from build123d import *

# Parameters (mm, degrees)
SKETCH_1_W          = 180
SKETCH_1_H          = 94
EXTRUDE_1_DEPTH     = 3
SKETCH_2_W          = 6
SKETCH_2_H          = 10
SKETCH_2_H_2        = 33.9
SKETCH_2_H_3        = 32.9
SKETCH_2_W_2        = 10
SKETCH_2_H_4        = 8
EXTRUDE_2_DEPTH     = 9
CHAMFER_2_SIZE      = 6
CHAMFER_1_SIZE      = 6
CUT_EXTRUDE_1_REACH = 205.421
SKETCH_3_R          = 1.5
SKETCH_3_R_2        = 1.75
SKETCH_4_R          = 1.5
CUT_EXTRUDE_2_DEPTH = 204.265835791
SKETCH_5_W          = 4
SKETCH_5_H          = 46
EXTRUDE_3_DEPTH     = 4
CHAMFER_3_SIZE      = 2
SKETCH_6_W          = 12
SKETCH_6_H          = 19.9
EXTRUDE_4_DEPTH     = 4
FILLET_1_R          = 4
SKETCH_7_W          = 12
SKETCH_7_H          = 19.9
EXTRUDE_5_DEPTH     = 4
FILLET_2_R          = 4
FILLET_3_R          = 2
SKETCH_8_R          = 1.5
CUT_EXTRUDE_3_DEPTH = 10
CUT_EXTRUDE_4_REACH = 208.969
SKETCH_9_R          = 1.5
CHAMFER_4_SIZE      = 6
FILLET_4_R          = 2


with BuildPart() as part:
    # Эскиз1 → Бобышка-Вытянуть1 (new body)
    with BuildSketch(Plane.XY):
        with Locations((90, -47)):
            Rectangle(SKETCH_1_W, SKETCH_1_H)
    extrude(amount=EXTRUDE_1_DEPTH)

    # Эскиз2 → Бобышка-Вытянуть2 (add)
    with BuildSketch(Plane.XY.offset(3)):
        with Locations((3, -89)):
            Rectangle(SKETCH_2_W, SKETCH_2_H)
        with Locations((177, -89)):
            Rectangle(SKETCH_2_W, SKETCH_2_H)
        with Locations((3, -52)):
            Rectangle(SKETCH_2_W, SKETCH_2_H)
        with Locations((177, -53)):
            Rectangle(SKETCH_2_W, SKETCH_2_H)
        with Locations((177, -25.05)):
            Rectangle(SKETCH_2_W, SKETCH_2_H_2)
        with Locations((3, -24.55)):
            Rectangle(SKETCH_2_W, SKETCH_2_H_3)
        with Locations((90.875995779, -90)):
            Rectangle(SKETCH_2_W_2, SKETCH_2_H_4)
    extrude(amount=EXTRUDE_2_DEPTH)

    # Фаска2
    chamfer_2_edges = [part.edges().sort_by_distance(p)[0] for p in [
        (3, -57, 3),
        (177, -58, 3),
    ]]
    chamfer(chamfer_2_edges, length=CHAMFER_2_SIZE)

    # Фаска1
    chamfer_1_edges = [part.edges().sort_by_distance(p)[0] for p in [
        (3, -84, 3),
        (177, -84, 3),
    ]]
    chamfer(chamfer_1_edges, length=CHAMFER_1_SIZE)

    # Эскиз3 → Вырез-Вытянуть1 (cut, up to next)
    with BuildSketch(Plane(origin=(180, 0, 0), x_dir=(0, 0, -1), z_dir=(1, 0, 0)), mode=Mode.PRIVATE) as cut_extrude_1_sk1:
        with Locations((-6, -89)):
            Circle(SKETCH_3_R)
    cut_extrude_1_tool1 = extrude(cut_extrude_1_sk1.sketch, amount=-CUT_EXTRUDE_1_REACH, mode=Mode.PRIVATE) & part.part
    # Эскиз3 → Вырез-Вытянуть1 (cut, up to next)
    with BuildSketch(Plane(origin=(180, 0, 0), x_dir=(0, 0, -1), z_dir=(1, 0, 0)), mode=Mode.PRIVATE) as cut_extrude_1_sk2:
        with Locations((-6, -53)):
            Circle(SKETCH_3_R)
    cut_extrude_1_tool2 = extrude(cut_extrude_1_sk2.sketch, amount=-CUT_EXTRUDE_1_REACH, mode=Mode.PRIVATE) & part.part
    # Эскиз3 → Вырез-Вытянуть1 (cut, up to next)
    with BuildSketch(Plane(origin=(180, 0, 0), x_dir=(0, 0, -1), z_dir=(1, 0, 0)), mode=Mode.PRIVATE) as cut_extrude_1_sk3:
        with Locations((-6, -34)):
            Circle(SKETCH_3_R_2)
    cut_extrude_1_tool3 = extrude(cut_extrude_1_sk3.sketch, amount=-CUT_EXTRUDE_1_REACH, mode=Mode.PRIVATE) & part.part
    add(cut_extrude_1_tool1.solids().sort_by_distance((180, -89, 6))[0], mode=Mode.SUBTRACT)
    add(cut_extrude_1_tool2.solids().sort_by_distance((180, -53, 6))[0], mode=Mode.SUBTRACT)
    add(cut_extrude_1_tool3.solids().sort_by_distance((180, -34, 6))[0], mode=Mode.SUBTRACT)

    # Эскиз4 → Вырез-Вытянуть2 (cut, through all)
    with BuildSketch(Plane.XY.offset(3)):
        with Locations((4, -4)):
            Circle(SKETCH_4_R)
        with Locations((176, -4)):
            Circle(SKETCH_4_R)
        with Locations((58, -4)):
            Circle(SKETCH_4_R)
        with Locations((122, -4)):
            Circle(SKETCH_4_R)
    extrude(amount=-CUT_EXTRUDE_2_DEPTH, mode=Mode.SUBTRACT)

    # Эскиз5 → Бобышка-Вытянуть3 (add)
    with BuildSketch(Plane.XY.offset(3)):
        with Locations((42, -71)):
            Rectangle(SKETCH_5_W, SKETCH_5_H)
        with Locations((138, -71)):
            Rectangle(SKETCH_5_W, SKETCH_5_H)
        Polygon((27, -4.5), (27, -37), (6, -37), (6, -41), (174, -41), (174, -37), (153, -37), (153, -4.5), (149, -4.5), (149, -37), (94, -37), (94, -4.5), (86, -4.5), (86, -37), (31, -37), (31, -4.5), align=None)
    extrude(amount=EXTRUDE_3_DEPTH)

    # Фаска3
    # the kernel refuses this chamfer: 2 mm, written as the material it adds along each edge
    with BuildSketch(Plane(origin=(6, -72.856634024, 3), x_dir=(0.9996219169112968, 0, -0.02749587661058627), z_dir=(0, -1, 0))) as chamfer_3_piece_1_section:
        Polygon((CHAMFER_3_SIZE * 0.999621916911, CHAMFER_3_SIZE * 0.0274958766106), (-CHAMFER_3_SIZE * 0.0274958766106, CHAMFER_3_SIZE * 0.999621916911), (0, 0), align=None)
    chamfer_3_piece_1 = extrude(amount=21.143365976, mode=Mode.PRIVATE)
    chamfer_3_piece_1 = split(chamfer_3_piece_1, bisect_by=Plane(origin=(6.668439358, -82.482271763, 7.482271763), z_dir=(0, -0.7071067811865476, -0.7071067811865476)), keep=Keep.TOP, mode=Mode.PRIVATE)
    add(chamfer_3_piece_1)
    with BuildSketch(Plane(origin=(174, -94, 3), x_dir=(-0.9996219169112968, 0, -0.02749587661058639), z_dir=(0, 1, 0))) as chamfer_3_piece_2_section:
        Polygon((CHAMFER_3_SIZE * 0.999621916911, CHAMFER_3_SIZE * 0.0274958766106), (-CHAMFER_3_SIZE * 0.0274958766106, CHAMFER_3_SIZE * 0.999621916911), (0, 0), align=None)
    chamfer_3_piece_2 = extrude(amount=21.143365976, mode=Mode.PRIVATE)
    chamfer_3_piece_2 = split(chamfer_3_piece_2, bisect_by=Plane(origin=(173.327651835, -82.469530213, 7.469530213), z_dir=(2.038461385028344e-15, -0.7071067811865476, -0.7071067811865476)), keep=Keep.TOP, mode=Mode.PRIVATE)
    chamfer_3_piece_2 = chamfer_3_piece_2 - Plane(origin=(173.327651835, -89, 6), x_dir=(0, 0, -1), z_dir=(1, 0, 0)) * Cylinder(1.5, 51, mode=Mode.PRIVATE)
    add(chamfer_3_piece_2)
    with BuildSketch(Plane(origin=(6, -47, 3), x_dir=(0.9996219169112968, 0, -0.02749587661058627), z_dir=(0, -1, 0))) as chamfer_3_piece_3_section:
        Polygon((CHAMFER_3_SIZE * 0.999621916911, CHAMFER_3_SIZE * 0.0274958766106), (-CHAMFER_3_SIZE * 0.0274958766106, CHAMFER_3_SIZE * 0.999621916911), (0, 0), align=None)
    chamfer_3_piece_3 = extrude(amount=21.143365976, mode=Mode.PRIVATE)
    chamfer_3_piece_3 = split(chamfer_3_piece_3, bisect_by=Plane(origin=(6.668439358, -58.517728237, 7.482271763), z_dir=(0, 0.7071067811865476, -0.7071067811865476)), keep=Keep.TOP, mode=Mode.PRIVATE)
    add(chamfer_3_piece_3)
    with BuildSketch(Plane(origin=(174, -69.143365976, 3), x_dir=(-0.9996219169112968, 0, -0.02749587661058639), z_dir=(0, 1, 0))) as chamfer_3_piece_4_section:
        Polygon((CHAMFER_3_SIZE * 0.999621916911, CHAMFER_3_SIZE * 0.0274958766106), (-CHAMFER_3_SIZE * 0.0274958766106, CHAMFER_3_SIZE * 0.999621916911), (0, 0), align=None)
    chamfer_3_piece_4 = extrude(amount=21.143365976, mode=Mode.PRIVATE)
    chamfer_3_piece_4 = split(chamfer_3_piece_4, bisect_by=Plane(origin=(173.327651834, -59.530469789, 7.469530211), z_dir=(0, 0.7071067811865476, -0.7071067811865476)), keep=Keep.TOP, mode=Mode.PRIVATE)
    chamfer_3_piece_4 = chamfer_3_piece_4 - Plane(origin=(173.327651834, -53, 6), x_dir=(0, 0, -1), z_dir=(1, 0, 0)) * Cylinder(1.5, 51, mode=Mode.PRIVATE)
    add(chamfer_3_piece_4)

    # Эскиз6 → Бобышка-Вытянуть4 (add)
    with BuildSketch(Plane(origin=(180, 0, 0), x_dir=(0, 0, -1), z_dir=(1, 0, 0))):
        with Locations((-6, -18.05)):
            Rectangle(SKETCH_6_W, SKETCH_6_H)
    extrude(amount=EXTRUDE_4_DEPTH)

    # Скругление1
    fillet_1_edges = [part.edges().sort_by_distance(p)[0] for p in [
        (184, -18.05, 12),
    ]]
    fillet(fillet_1_edges, radius=FILLET_1_R)

    # Эскиз7 → Бобышка-Вытянуть5 (add)
    with BuildSketch(Plane.ZY):
        with Locations((6, -18.05)):
            Rectangle(SKETCH_7_W, SKETCH_7_H)
    extrude(amount=EXTRUDE_5_DEPTH)

    # Скругление2
    fillet_2_edges = [part.edges().sort_by_distance(p)[0] for p in [
        (-4, -18.05, 12),
    ]]
    fillet(fillet_2_edges, radius=FILLET_2_R)

    # Скругление3
    fillet_3_edges = [part.edges().sort_by_distance(p)[0] for p in [
        (184, -18.05, 0),
        (-4, -18.05, 0),
    ]]
    fillet(fillet_3_edges, radius=FILLET_3_R)

    # Эскиз8 → Вырез-Вытянуть3 (cut)
    with BuildSketch(Plane.XZ.offset(94)):
        with Locations(Location((90.875995779, 8, 0), (0, 0, 270))):
            Circle(SKETCH_8_R)
    extrude(amount=-CUT_EXTRUDE_3_DEPTH, mode=Mode.SUBTRACT)

    # Эскиз9 → Вырез-Вытянуть4 (cut, up to next)
    with BuildSketch(Plane.ZY, mode=Mode.PRIVATE) as cut_extrude_4_sk1:
        with Locations(Location((6, -89, 0), (0, 0, 180))):
            Circle(SKETCH_9_R)
    cut_extrude_4_tool1 = extrude(cut_extrude_4_sk1.sketch, amount=-CUT_EXTRUDE_4_REACH, mode=Mode.PRIVATE) & part.part
    # Эскиз9 → Вырез-Вытянуть4 (cut, up to next)
    with BuildSketch(Plane.ZY, mode=Mode.PRIVATE) as cut_extrude_4_sk2:
        with Locations(Location((6, -53, 0), (0, 0, 180))):
            Circle(SKETCH_9_R)
    cut_extrude_4_tool2 = extrude(cut_extrude_4_sk2.sketch, amount=-CUT_EXTRUDE_4_REACH, mode=Mode.PRIVATE) & part.part
    add(cut_extrude_4_tool1.solids().sort_by_distance((0, -89, 6))[0], mode=Mode.SUBTRACT)
    add(cut_extrude_4_tool2.solids().sort_by_distance((0, -53, 6))[0], mode=Mode.SUBTRACT)

    # Фаска4
    chamfer_4_edges = [part.edges().sort_by_distance(p)[0] for p in [
        (85.875995779, -90, 3),
        (95.875995779, -90, 3),
    ]]
    chamfer(chamfer_4_edges, length=CHAMFER_4_SIZE)

    # Скругление4
    fillet_4_edges = [part.edges().sort_by_distance(p)[0] for p in [
        (177, -84, 12),
        (3, -84, 12),
        (3, -41, 12),
        (3, -47, 12),
        (3, -57, 12),
        (3, -94, 12),
        (177, -42, 12),
        (177, -48, 12),
        (177, -58, 12),
        (85.875995779, -90, 12),
        (95.875995779, -90, 12),
        (177, -94, 12),
    ]]
    fillet(fillet_4_edges, radius=FILLET_4_R)


solid = part.part
Check sheet for the modelled part. Datum: model origin and axes. Units: mm. A direction names the side the tool comes from. Coordinates: 2 decimals unless noted, no trailing zeros. Loops run counter-clockwise (first coordinate to the right, second up) from the corner with the lowest first, then second, coordinate; pieces in that order, holes last. Notation, with made-up numbers: (7, 64) -> (62, 64) arc R27 ccw to (62, 98) -> close; hole circle Ø2 at (-17, -9). An arc over 180 degrees is marked (long way). Write item = value, one per line. Start each with the question number.
1. Depth check by flat-ended pin: P1, Ø3, axis at y = -80, z = 4.5, coming from the +X side; P2, Ø0.8, axis at x = 177, z = 9.5, coming from the +Y side; P3, Ø1.5, axis at x = 152, y = -65, coming from the +Z side. Enter the tip coordinate at first touch or a pass-through.
2. Tool access check on faces 4 (the flat face through (138, -71, 7)), 5 (the flat face through (6, -25, 7)), 6 (the flat face through (174, -54, 8)). Record the directions out of +Z, -Z, +X, -X, +Y, -Y that give a thin tool (end or side, any length) a straight path to the whole face; none if there is none.
3. Section check B-B on y = -12. Record the cut outline in (x, z).
4. Draft check along X on faces 1 (the flat face through (0, -61, 3)), 2 (the flat face through (177, -81, 6)), 3 (the flat face through (82.918, -90.056, 6.042)). Enter one of: released by +X, released by -X, zero draft, split by the parting line, or undercut.
5. Section check A-A on y = -34. Record the cut outline in (x, z), then the cut area to 3 significant figures.
6. Material ranges on line 1 (X direction, y = -20, z = 5.75); line 2 (Y direction, x = 122, z = 2.3); line 3 (Y direction, x = 177, z = 6), recorded low to high.
7. Section check C-C on x = 113. Record the cut outline in (y, z), then the cut area to 3 significant figures.
Responses:
q1.P1 = 180
q1.P2 = -8.1
q1.P3 = 3
q2.face_4 = +Z, +Y, -Y
q2.face_5 = +Z, +Y
q2.face_6 = +Z, -Y
q3.outline = (-4, 2) arc R2 ccw to (-2, 0) -> (182, 0) arc R2 ccw to (184, 2) -> (184, 8) arc R4 ccw to (180, 12) -> (174, 12) -> (174, 3) -> (153, 3) -> (153, 7) -> (149, 7) -> (149, 3) -> (94, 3) -> (94, 7) -> (86, 7) -> (86, 3) -> (31, 3) -> (31, 7) -> (27, 7) -> (27, 3) -> (6, 3) -> (6, 12) -> (0, 12) arc R4 ccw to (-4, 8) -> close
q4.face_1 = released by -X
q4.face_2 = zero draft
q4.face_3 = undercut
q5.outline = (0, 0) -> (180, 0) -> (180, 4.25) -> (174, 4.25) -> (174, 3) -> (153, 3) -> (153, 7) -> (149, 7) -> (149, 3) -> (94, 3) -> (94, 7) -> (86, 7) -> (86, 3) -> (31, 3) -> (31, 7) -> (27, 7) -> (27, 3) -> (6, 3) -> (6, 12) -> (0, 12) -> close; (174, 7.75) -> (180, 7.75) -> (180, 12) -> (174, 12) -> close
q5.area = 691 mm2
q6.line_1 = -4 to 6, 27 to 31, 86 to 94, 149 to 153, 174 to 184
q6.line_2 = -94 to -5.5, -2.5 to 0
q6.line_3 = -94 to -90.5, -87.5 to -81, -61 to -54.5, -51.5 to -48, -42 to -35.75, -32.25 to -8.1
q7.outline = (-94, 0) -> (0, 0) -> (0, 3) -> (-37, 3) -> (-37, 7) -> (-41, 7) -> (-41, 3) -> (-94, 3) -> close
q7.area = 298 mm2
